Verification items for the finished model (mm, model axes). A direction names the side the tool comes from. Round coordinates to 2 decimals unless told otherwise and drop trailing zeros. Order: outer loops, then holes, each group sorted by start corner. A loop starts at its lowest first (then second) coordinate and runs counter-clockwise, first axis right, second up. Notation, with made-up numbers: M -12.75,-18.75 L -3.75,-18.75 A10 ccw -3.75,-3.75 Z; hole C 75.5,-10.75 d10. An arc over 180 degrees is marked long. Write item = value, one per line. Start each with the question number.
from build123d import *

# Parameters (mm, degrees)
BOSS_EXTRUDE1_DEPTH = 50.8
SKETCH3_W           = 25.4
SKETCH3_H           = 25.4
CUT_EXTRUDE1_DEPTH  = 25.4
SKETCH8_W           = 24.892
SKETCH8_H           = 24.892
BOSS_EXTRUDE2_DEPTH = 24.892
SKETCH12_R          = 3.429
CUT_EXTRUDE2_DEPTH  = 25.4
SKETCH13_W          = 25.4
SKETCH13_H          = 12.7
CUT_EXTRUDE3_DEPTH  = 25.908
FILLET1_R           = 2.54
SKETCH14_R          = 3.175
CUT_EXTRUDE5_DEPTH  = 246.663470197
CUT_EXTRUDE6_DEPTH  = 5.08
SKETCH18_W          = 91.44
SKETCH18_H          = 43.18
CUT_EXTRUDE7_DEPTH  = 7.62


with BuildPart() as part:
    # Sketch2 → Boss-Extrude1 (new body)
    with BuildSketch(Plane(origin=(0, 0, 0), x_dir=(1, 0, 0), z_dir=(0, 1, 0))):
        Polygon((-50.8, 155.575), (0, 155.575), (0, 0), (107.95, 0), (107.95, -50.8), (-50.8, -50.8), align=None)
    extrude(amount=BOSS_EXTRUDE1_DEPTH)

    # Sketch3 → Cut-Extrude1 (cut)
    with BuildSketch(Plane(origin=(107.95, 0, 0), x_dir=(0, 0, -1), z_dir=(1, 0, 0))):
        with Locations((-25.239912, 25.560088)):
            Rectangle(SKETCH3_W, SKETCH3_H)
    extrude(amount=-CUT_EXTRUDE1_DEPTH, mode=Mode.SUBTRACT)

    # Sketch7 → CBORE for 1/4 Binding Head Machine Screw1 (revolve, cut)
    with BuildSketch(Plane(origin=(95.25, 50.8, 25.4), x_dir=(0, 0, 1), z_dir=(1, 0, 0))):
        Polygon((0, 0), (0, 50.8), (3.3782, 50.8), (3.3782, 4.191), (7.14375, 4.191), (7.14375, 0.635), (7.77875, 0), align=None)
    revolve(axis=Axis((95.25, 57.15, 25.4), (0, -1, 0)), mode=Mode.SUBTRACT)

    # Sketch8 → Boss-Extrude2 (add)
    with BuildSketch(Plane(origin=(0, 0, -155.575), x_dir=(-1, 0, 0), z_dir=(0, 0, -1))):
        with Locations((25.4, 25.4)):
            Rectangle(SKETCH8_W, SKETCH8_H)
    extrude(amount=BOSS_EXTRUDE2_DEPTH)

    # Sketch12 → Cut-Extrude2 (cut)
    with BuildSketch(Plane(origin=(0, 37.846, 0), x_dir=(1, 0, 0), z_dir=(0, 1, 0))):
        with Locations(Location((-25.4, 168.275, 0), (0, 0, 270))):
            Circle(SKETCH12_R)
    extrude(amount=-CUT_EXTRUDE2_DEPTH, mode=Mode.SUBTRACT)

    # Sketch13 → Cut-Extrude3 (cut)
    with BuildSketch(Plane(origin=(0, 50.8, 0), x_dir=(1, 0, 0), z_dir=(0, 1, 0))):
        with Locations((-25.4, 117.475)):
            Rectangle(SKETCH13_W, SKETCH13_H)
    extrude(amount=-CUT_EXTRUDE3_DEPTH, mode=Mode.SUBTRACT)

    # Fillet1
    fillet1_edges = [part.edges().sort_by_distance(p)[0] for p in [
        (-38.1, 50.8, -117.475),
        (-12.7, 50.8, -117.475),
    ]]
    fillet(fillet1_edges, radius=FILLET1_R)

    # Sketch14 → Cut-Extrude5 (cut, through all)
    with BuildSketch(Plane.ZY.offset(50.8)):
        with Locations((-117.475, 38.1)):
            Circle(SKETCH14_R)
    extrude(amount=-CUT_EXTRUDE5_DEPTH, mode=Mode.SUBTRACT)

    # Sketch17 → Cut-Extrude6 (cut)
    with BuildSketch(Plane(origin=(0, 50.8, 0), x_dir=(1, 0, 0), z_dir=(0, 1, 0))):
        Polygon((0, 155.575), (0, 0), (107.95, 0), (107.95, -7.62), (-7.62, -7.62), (-7.62, 155.575), align=None)
    extrude(amount=-CUT_EXTRUDE6_DEPTH, mode=Mode.SUBTRACT)

    # Sketch18 → Cut-Extrude7 (cut)
    with BuildSketch(Plane(origin=(0, 50.8, 0), x_dir=(1, 0, 0), z_dir=(0, 1, 0))):
        with Locations((38.1, -29.21)):
            Rectangle(SKETCH18_W, SKETCH18_H)
    extrude(amount=-CUT_EXTRUDE7_DEPTH, mode=Mode.SUBTRACT)


solid = part.part
1) Cross-section at C-C, the plane z = 25.4. Enter the section's corners in (x, y) (3 decimals), then the cut area to 3 significant figures.
2) Cross-section at D-D, the plane z = -9. Enter the section's corners in (x, y).
3) Scan lines: probe 1 along X at (y, z) = (48, 25); probe 2 along X at (y, z) = (7, 25); probe 3 along Z at (x, y) = (95.25, 3). Record each from-to range of solid material in increasing order.
4) Cross-section at A-A, the plane x = -25.4. Enter the section's corners in (y, z) (3 decimals), then the cut area to 3 significant figures.
5) Release check for a two-part mould opening along X. For faces 5 (the flat face through (-12.954, 25, -168)), 6 (the flat face through (-7.62, 48, -51)), 7 (the flat face through (-29, 50.8, -54)) record: pulls with the +X half, pulls with the -X half, needs draft (parallel to the pull), parting line crosses it, or undercut.
6) Cross-section at B-B, the plane y = 28.5. Enter the section's corners in (x, z) (3 decimals), then the cut area to 3 significant figures.
7) Access from +Z, -Z, +X, -X, +Y, -Y to the whole of each face (thin tool, end or side, straight path). Record for faces 1 (the flat face through (-26, 38, -111.125)), 2 (the flat face through (-37.846, 25, -168)), 3 (the flat face through (-28, 37.846, -171)), 4 (the flat face through (96, 48, 7.62)).
8) Gauge pin test, flat ends, axial feed: P1, Ø14, axis at y = 37, z = -116.5, coming from the +X side; P2, Ø10, axis at x = 67, z = 22, coming from the +Y side; P3, Ø6, axis at x = 72, y = 38.5, coming from the -Z side. Record the tip position at first contact, or that the pin passes through.
Geometry results:
q1.outline = M -50.8,0 L 91.872,0 L 91.872,12.86 L 82.55,12.86 L 82.55,38.26 L 91.872,38.26 L 91.872,46.609 L 88.106,46.609 L 88.106,50.165 L 87.471,50.8 L 83.82,50.8 L 83.82,43.18 L -7.62,43.18 L -7.62,50.8 L -50.8,50.8 Z; M 98.628,0 L 107.95,0 L 107.95,12.86 L 98.628,12.86 Z; M 98.628,38.26 L 107.95,38.26 L 107.95,50.8 L 103.029,50.8 L 102.394,50.165 L 102.394,46.609 L 98.628,46.609 Z
q1.area = 6,520 mm^2
q2.outline = M -50.8,0 L 0,0 L 0,45.72 L -7.62,45.72 L -7.62,50.8 L -50.8,50.8 Z
q3.probe_1 = -50.8 to -7.62, 83.82 to 88.12, 102.38 to 107.95
q3.probe_2 = -50.8 to 91.9, 98.6 to 107.95
q3.probe_3 = 0 to 22.02, 28.78 to 50.8
q4.outline = M 0,-155.575 L 12.954,-155.575 L 12.954,-164.846 L 37.846,-164.846 L 37.846,-155.575 L 50.8,-155.575 L 50.8,-123.825 L 24.892,-123.825 L 24.892,-111.125 L 50.8,-111.125 L 50.8,50.8 L 0,50.8 Z; M 12.954,-180.467 L 37.846,-180.467 L 37.846,-171.704 L 12.954,-171.704 Z
q4.area = 10,600 mm^2
q5.face_5 = pulls with the +X half
q5.face_6 = undercut
q5.face_7 = needs draft
q6.outline = M -50.8,-155.575 L -37.846,-155.575 L -37.846,-180.467 L -12.954,-180.467 L -12.954,-155.575 L 0,-155.575 L 0,0 L 107.95,0 L 107.95,12.54 L 82.55,12.54 L 82.55,37.94 L 107.95,37.94 L 107.95,50.8 L -50.8,50.8 Z; hole M -38.1,-123.825 L -12.7,-123.825 L -12.7,-111.125 L -38.1,-111.125 Z; hole C -25.4,-168.275 d6.858
q6.area = 15,600 mm^2
q7.face_1 = +Y
q7.face_2 = -Z, -X, +Y, -Y
q7.face_3 = -Z, +X, -X, +Y
q7.face_4 = -Z, +X, +Y
q8.P1 = 0
q8.P2 = 43.18
q8.P3 = 0
